Geometry check sheet. Reference: drawing and pictorial views, mm from the part's lowest x, y, z. A direction names the side the tool comes from. Round coordinates to 2 decimals unless told otherwise and drop trailing zeros. Order: outer loops, then holes, each group sorted by start corner. A loop starts at its lowest first (then second) coordinate and runs counter-clockwise, first axis right, second up.
(1) Thickness scan on L1, parallel to Z at x = 9.75, y = 6.25; L2, parallel to Y at x = 8, z = 3.4; L3, parallel to Y at x = 5.25, z = 4.3. Record the ranges inside material, lowest first.
(2) Cross-section at A-A on x = 4.75. Enter the section's corners in (y, z).
(3) Cross-section at C-C on z = 1.55. Enter the section's corners in (x, y).
(4) Gauge pin test, flat ends, axial feed: P1, Ø1.8, axis at x = 4, y = 1, coming from the +Z side; P2, Ø0.8, axis at x = 6.5, y = 3, coming from the -Z side; P3, Ø1.8, axis at x = 9.91, z = 3, coming from the -Y side; P4, Ø2, axis at y = 4, z = 1.5, coming from the +X side. Record the tip position at first contact, or that the pin passes through.
(5) Set-up check for the marked faces 1, 2 and 3: record each of +Z, -Z, +X, -X, +Y, -Y from which the full face is reachable in a straight line by a thin tool's end or side.
(6) Cross-section at B-B on y = 4. Enter the section's corners in (x, z).
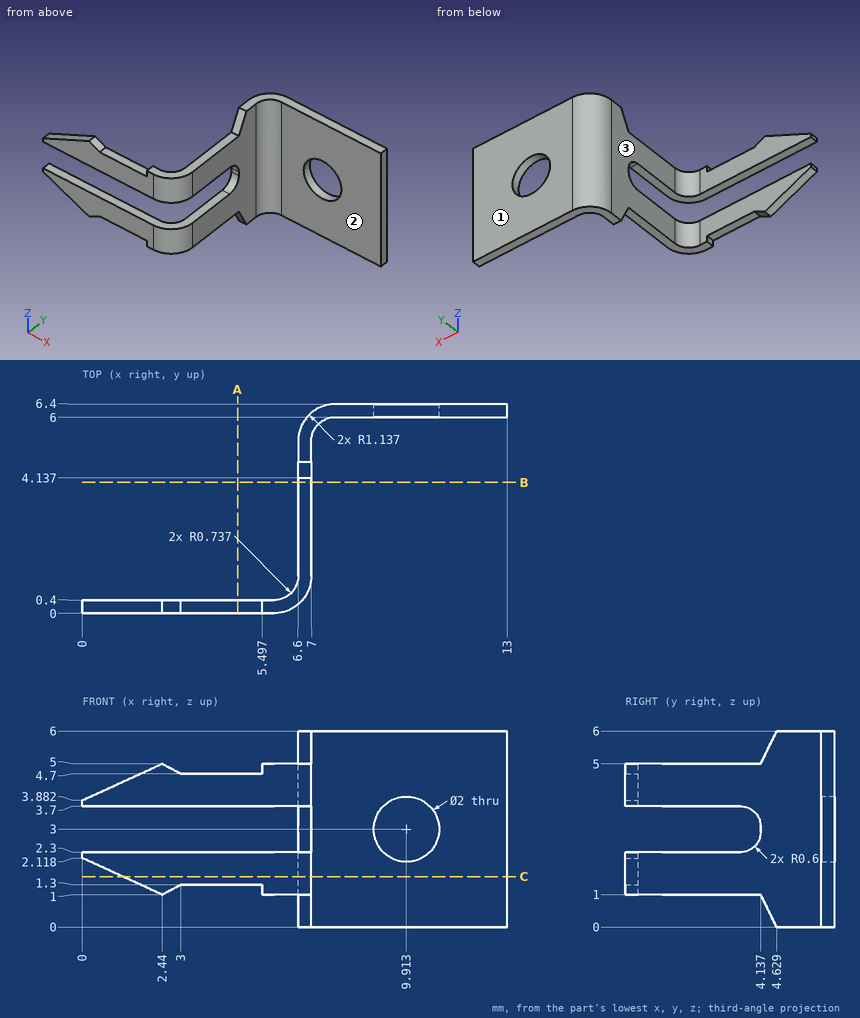
Found:
1. L1: z = 0 to 2.01, 3.99 to 6
1. L2: y = 6 to 6.4
1. L3: y = 0 to 0.4
2. outline: (0, 1.3) - (0.4, 1.3) - (0.4, 2.3) - (0, 2.3) - close; (0, 3.7) - (0.4, 3.7) - (0.4, 4.7) - (0, 4.7) - close
3. outline: (1.24, 0) - (5.86, 0) arc R1.14 ccw to (7, 1.14) - (7, 5.26) arc R0.74 cw to (7.74, 6) - (13, 6) - (13, 6.4) - (7.74, 6.4) arc R1.14 ccw to (6.6, 5.26) - (6.6, 1.14) arc R0.74 cw to (5.86, 0.4) - (1.24, 0.4) - close
4. P1: stops at z = 4.7
4. P2: stops at z = 1
4. P3: passes through
4. P4: stops at x = 7
5. face 1: +Z, -Z, +X, -X, +Y
5. face 2: +Z, -Z, +X, -Y
5. face 3: +Z, -Z, -X, +Y
6. outline: (6.6, 1) - (7, 1) - (7, 2.52) - (6.6, 2.52) - close; (6.6, 3.48) - (7, 3.48) - (7, 5) - (6.6, 5) - close
